```python
from build123d import *

# Parameters (mm, degrees)
SKETCH1_R           = 6
BOSS_EXTRUDE1_DEPTH = 28
CUT_EXTRUDE1_START  = -15.5
CUT_EXTRUDE1_DEPTH  = 15.5
CUT_EXTRUDE2_DEPTH  = 31.01666204
SKETCH4_R           = 2.5
CUT_EXTRUDE3_DEPTH  = 31.01666204
FILLET1_R           = 1
CUT_EXTRUDE4_DEPTH  = 31.016662183
SKETCH7_R           = 2.5
CUT_EXTRUDE5_DEPTH  = 10


with BuildPart() as part:
    # Sketch1 → Boss-Extrude1 (new body)
    with BuildSketch(Plane(origin=(0, 0, 0), x_dir=(1, 0, 0), z_dir=(0, 1, 0))):
        with Locations(Location((0, 0, 0), (0, 0, 270))):
            Circle(SKETCH1_R)
    extrude(amount=BOSS_EXTRUDE1_DEPTH)

    # Sketch2 → Cut-Extrude1 (cut)
    with BuildSketch(Plane(origin=(0, 28, 0), x_dir=(1, 0, 0), z_dir=(0, 1, 0)).offset(CUT_EXTRUDE1_START)):
        with BuildLine():
            ThreePointArc((5.196152423, 3), (0, 6), (-5.196152423, 3))
            Line((-5.196152423, 3), (5.196152423, 3))
        make_face()
        with BuildLine():
            Line((5.196152423, -3), (-5.196152423, -3))
            ThreePointArc((-5.196152423, -3), (0, -6), (5.196152423, -3))
        make_face()
    extrude(amount=CUT_EXTRUDE1_DEPTH, mode=Mode.SUBTRACT)

    # Sketch3 → Cut-Extrude2 (cut, through all)
    with BuildSketch(Plane.XY.offset(3)):
        with BuildLine():
            ThreePointArc((-5.196152423, 25), (-3, 27.196152423), (0, 28))
            Line((0, 28), (-5.196152423, 28))
            Line((-5.196152423, 28), (-5.196152423, 25))
        make_face()
        with BuildLine():
            ThreePointArc((0, 28), (3, 27.196152423), (5.196152423, 25))
            Line((5.196152423, 25), (5.196152423, 28))
            Line((5.196152423, 28), (0, 28))
        make_face()
    extrude(amount=-CUT_EXTRUDE2_DEPTH, mode=Mode.SUBTRACT)

    # Sketch4 → Cut-Extrude3 (cut, through all)
    with BuildSketch(Plane.XY.offset(3)):
        with Locations((0, 22)):
            Circle(SKETCH4_R)
    extrude(amount=-CUT_EXTRUDE3_DEPTH, mode=Mode.SUBTRACT)

    # Fillet1
    fillet1_edges = [part.edges().sort_by_distance(p)[0] for p in [
        (0, 12.5, -3),
        (0, 12.5, 3),
    ]]
    fillet(fillet1_edges, radius=FILLET1_R)

    # Sketch6 → Cut-Extrude4 (cut, through all)
    with BuildSketch(Plane.XY.offset(3)):
        with BuildLine():
            Line((-6, 28), (-6, 22))
            ThreePointArc((-6, 22), (-5.795554958, 23.552914271), (-5.196152423, 25))
            ThreePointArc((-5.196152423, 25), (-3, 27.196152423), (0, 28))
            Line((0, 28), (-6, 28))
        make_face()
        with BuildLine():
            ThreePointArc((5.196152423, 25), (5.795554958, 23.552914271), (6, 22))
            Line((6, 22), (6, 28))
            Line((6, 28), (0, 28))
            ThreePointArc((0, 28), (3, 27.196152423), (5.196152423, 25))
        make_face()
    extrude(amount=-CUT_EXTRUDE4_DEPTH, mode=Mode.SUBTRACT)

    # Sketch7 → Cut-Extrude5 (cut)
    with BuildSketch(Plane.XZ):
        with Locations(Location((0, 0, 0), (0, 0, 270))):
            Circle(SKETCH7_R)
    extrude(amount=-CUT_EXTRUDE5_DEPTH, mode=Mode.SUBTRACT)


solid = part.part
```
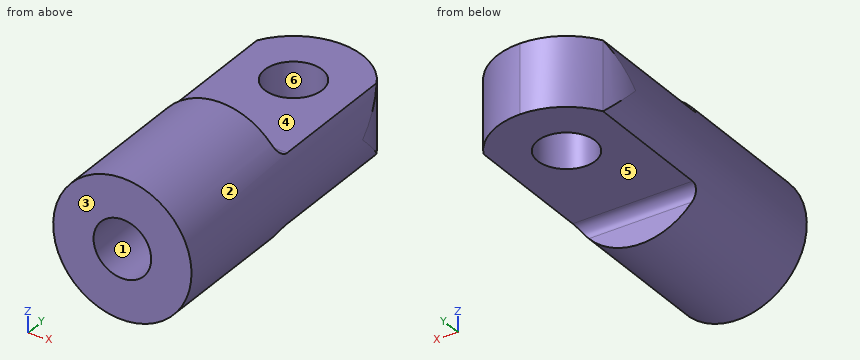
Check sheet for the modelled part. Datum: model origin and axes. Units: mm. Face numbers are marked on the shaded views. A direction names the side the tool comes from. Round coordinates to 2 decimals unless told otherwise and drop trailing zeros. Loops run counter-clockwise (first coordinate to the right, second up) from the corner with the lowest first, then second, coordinate; pieces in that order, holes last. Notation, with made-up numbers: M -2,82.5 L 38,82.5 A10 cw 38,87.5 Z; hole C 56,-13.75 d1. An arc over 180 degrees is marked long. Answer as a JSON object with one key per item and string values.
1. Scan lines: line 1 (X direction, y = 3, z = 0); line 2 (X direction, y = 11.5, z = -0.25); line 3 (Y direction, x = 0.5, z = -1.5). Record each from-to range of solid material in increasing order.
Reply:
{"line 1": "x = -6 to -2.5, 2.5 to 6", "line 2": "x = -5.99 to 5.99", "line 3": "y = 10 to 19.55, 24.45 to 27.98"}
2. Access from +Z, -Z, +X, -X, +Y, -Y to the whole of each face (thin tool, end or side, straight path). Record for the marked faces 4, 5 and 6.
Reply:
{"face 4": "+Z, +X, -X, +Y", "face 5": "-Z, +X, -X, +Y", "face 6": "+Z, -Z"}
3. Mould release check, pull along X, two halves, no side actions. Record for the marked faces 1, 2 and 3: pulls with the +X half, pulls with the -X half, needs draft (parallel to the pull), parting line crosses it, or undercut.
Reply:
{"face 1": "undercut", "face 2": "parting line crosses it", "face 3": "needs draft"}
4. Gauge pin test, flat ends, axial feed: P1, Ø2, axis at x = -1.5, z = -5.5, coming from the +Y side; P2, Ø3, axis at x = 4.5, y = 15.5, coming from the -Z side; P3, Ø4.5, axis at x = 0, y = 22, coming from the +Z side; P4, Ø1.5, axis at y = 3.5, z = -5, coming from the +X side. Record the tip position at first contact, or that the pin passes through.
Reply:
{"P1": "stops at y = 12.5", "P2": "stops at z = -3", "P3": "passes through", "P4": "stops at x = 4.24"}
5. Section check B-B (y = 24). Record the boundary of the cut face in (x, z), plus the area to 3 significant figures.
Reply:
{"outline": "M -5.66,-2 A6 ccw -5.2,-3 L -1.5,-3 L -1.5,3 L -5.2,3 A6 ccw -5.66,2 Z; M 1.5,-3 L 5.2,-3 A6 ccw 5.66,-2 L 5.66,2 A6 ccw 5.2,3 L 1.5,3 Z", "area": "49.0 mm²"}
6. Section check A-A (z = 0). Record the boundary of the cut face in (x, y), plus the area to 3 significant figures.
Reply:
{"outline": "M -6,0 L -2.5,0 L -2.5,10 L 2.5,10 L 2.5,0 L 6,0 L 6,22 A6 ccw -6,22 Z; hole C 0,22 d5", "area": "251 mm²"}
7. Section check C-C (x = -3.75). Record the boundary of the cut face in (y, z), plus the area to 3 significant figures.
Reply:
{"outline": "M 0,-4.68 L 12.5,-4.68 L 12.5,-4 A1 cw 13.5,-3 L 26.68,-3 L 26.68,3 L 13.5,3 A1 cw 12.5,4 L 12.5,4.68 L 0,4.68 Z", "area": "203 mm²"}
8. Section check D-D (y = 3.75). Record the boundary of the cut face in (x, z).
Reply:
{"outline": "C 0,0 d12; hole C 0,0 d5"}
